```python
from build123d import *

# Parameters (mm, degrees)
BOSS_EXTRU_1_DEPTH      = 24
ESQUISSE2_W             = 2
ESQUISSE2_H             = 0.5
BOSS_EXTRU_2_DEPTH      = 3
BOSS_EXTRU_3_DEPTH      = 3
ESQUISSE6_W             = 0.6
ESQUISSE6_H             = 2
ENL_V_MAT_EXTRU_1_DEPTH = 1.5
BOSS_EXTRU_4_DEPTH      = 4
ENL_V_MAT_EXTRU_3_REACH = 29.975
ESQUISSE8_R             = 0.5
ESQUISSE9_W             = 0.5
ESQUISSE9_H             = 2
BOSS_EXTRU_5_DEPTH      = 3
ENL_V_MAT_EXTRU_2_REACH = 30.233
ESQUISSE7_R             = 0.35


with BuildPart() as part:
    # Esquisse1 → Boss.-Extru.1 (new body)
    with BuildSketch(Plane.XY):
        with BuildLine():
            Line((-3, 7), (3, 7))
            ThreePointArc((3, 7), (3.424264069, 6.824264069), (3.6, 6.4))
            Line((3.6, 6.4), (3.6, 0))
            Line((3.6, 0), (3.1, 0))
            Line((3.1, 0), (3.1, 6.4))
            ThreePointArc((3.1, 6.4), (3.070710678, 6.470710678), (3, 6.5))
            Line((3, 6.5), (-3, 6.5))
            ThreePointArc((-3, 6.5), (-3.070710678, 6.470710678), (-3.1, 6.4))
            Line((-3.1, 6.4), (-3.1, 0))
            Line((-3.1, 0), (-3.6, 0))
            Line((-3.6, 0), (-3.6, 6.4))
            ThreePointArc((-3.6, 6.4), (-3.424264069, 6.824264069), (-3, 7))
        make_face()
    extrude(amount=BOSS_EXTRU_1_DEPTH)

    # Esquisse2 → Boss.-Extru.2 (add)
    with BuildSketch(Plane(origin=(0, 0, 0), x_dir=(-1, 0, 0), z_dir=(0, 0, -1))):
        with Locations((0, 6.75)):
            Rectangle(ESQUISSE2_W, ESQUISSE2_H)
    extrude(amount=BOSS_EXTRU_2_DEPTH)

    # Esquisse5 → Boss.-Extru.3 (add)
    with BuildSketch(Plane.ZY.offset(1)):
        with BuildLine():
            Line((-0.1, 1), (-0.6, 1))
            Line((-0.6, 1), (-0.6, 6.4))
            ThreePointArc((-0.6, 6.4), (-0.424264069, 6.824264069), (0, 7))
            Line((0, 7), (0, 6.5))
            ThreePointArc((0, 6.5), (-0.070710678, 6.470710678), (-0.1, 6.4))
            Line((-0.1, 6.4), (-0.1, 1))
        make_face()
    boss_extru_3 = extrude(amount=BOSS_EXTRU_3_DEPTH)

    # Esquisse6 → Enl_v. mat.-Extru.1 (cut)
    with BuildSketch(Plane.ZY.offset(4)):
        with Locations((-0.3, 6)):
            Rectangle(ESQUISSE6_W, ESQUISSE6_H)
    enl_v_mat_extru_1 = extrude(amount=-ENL_V_MAT_EXTRU_1_DEPTH, mode=Mode.SUBTRACT)

    # Esquisse3 → Boss.-Extru.4 (add)
    with BuildSketch(Plane(origin=(0, 5, 0), x_dir=(1, 0, 0), z_dir=(0, 1, 0))):
        with BuildLine():
            Line((-4.491491227, 0.344145862), (-9.653679154, -7.028222537))
            Line((-9.653679154, -7.028222537), (-9.244103132, -7.315010755))
            Line((-9.244103132, -7.315010755), (-4.081915204, 0.057357644))
            ThreePointArc((-4.081915204, 0.057357644), (-4.046174861, 0.088701083), (-4, 0.1))
            Line((-4, 0.1), (-4, 0.6))
            ThreePointArc((-4, 0.6), (-4.277049168, 0.5322065), (-4.491491227, 0.344145862))
        make_face()
    boss_extru_4 = extrude(amount=-BOSS_EXTRU_4_DEPTH)

    # Esquisse8 → Enl_v. mat.-Extru.3 (cut, up to next)
    with BuildSketch(Plane(origin=(-3.175531513, 0, -2.223531103), x_dir=(-0.5735764363510417, 0, 0.8191520442889949), z_dir=(-0.819152044288995, 0, -0.5735764363510417)), mode=Mode.PRIVATE) as enl_v_mat_extru_3_sk1:
        with Locations((8.058237768, 3)):
            Circle(ESQUISSE8_R)
    enl_v_mat_extru_3_tool1 = extrude(enl_v_mat_extru_3_sk1.sketch, amount=-ENL_V_MAT_EXTRU_3_REACH, mode=Mode.PRIVATE) & part.part
    # Esquisse8 → Enl_v. mat.-Extru.3 (cut, up to next)
    with BuildSketch(Plane(origin=(-3.175531513, 0, -2.223531103), x_dir=(-0.5735764363510417, 0, 0.8191520442889949), z_dir=(-0.819152044288995, 0, -0.5735764363510417)), mode=Mode.PRIVATE) as enl_v_mat_extru_3_sk2:
        with BuildLine():
            Line((11.294305745, 1), (10.294305745, 1))
            ThreePointArc((10.294305745, 1), (11.058237768, 3), (10.294305745, 5))
            Line((10.294305745, 5), (11.294305745, 5))
            Line((11.294305745, 5), (11.294305745, 1))
        make_face()
    enl_v_mat_extru_3_tool2 = extrude(enl_v_mat_extru_3_sk2.sketch, amount=-ENL_V_MAT_EXTRU_3_REACH, mode=Mode.PRIVATE) & part.part
    enl_v_mat_extru_3_1 = enl_v_mat_extru_3_tool1.solids().sort_by_distance((-7.797547, 3, 4.377391))[0]
    add(enl_v_mat_extru_3_1, mode=Mode.SUBTRACT)
    enl_v_mat_extru_3_2 = enl_v_mat_extru_3_tool2.solids().sort_by_distance((-9.541925, 3, 6.868621))[0]
    add(enl_v_mat_extru_3_2, mode=Mode.SUBTRACT)
    enl_v_mat_extru_3 = enl_v_mat_extru_3_1 + enl_v_mat_extru_3_2  # Enl_v. mat.-Extru.3 as one shape, for the pattern or mirror that repeats it

    # Esquisse9 → Boss.-Extru.5 (add)
    with BuildSketch(Plane.XZ):
        with Locations((-3.35, 7.5)):
            Rectangle(ESQUISSE9_W, ESQUISSE9_H)
        with Locations((-3.35, 20.5)):
            Rectangle(ESQUISSE9_W, ESQUISSE9_H)
    boss_extru_5 = extrude(amount=BOSS_EXTRU_5_DEPTH)

    # Sym_trie1: Boss.-Extru.3, Enl_v. mat.-Extru.1, Boss.-Extru.4, Enl_v. mat.-Extru.3, Boss.-Extru.5 across plane
    add(boss_extru_3.mirror(Plane(origin=(0, 0, 0), x_dir=(0, 0, 1), z_dir=(1, 0, 0))))
    add(enl_v_mat_extru_1.mirror(Plane(origin=(0, 0, 0), x_dir=(0, 0, 1), z_dir=(1, 0, 0))), mode=Mode.SUBTRACT)
    add(boss_extru_4.mirror(Plane(origin=(0, 0, 0), x_dir=(0, 0, 1), z_dir=(1, 0, 0))))
    add(enl_v_mat_extru_3.mirror(Plane(origin=(0, 0, 0), x_dir=(0, 0, 1), z_dir=(1, 0, 0))), mode=Mode.SUBTRACT)
    add(boss_extru_5.mirror(Plane(origin=(0, 0, 0), x_dir=(0, 0, 1), z_dir=(1, 0, 0))))

    # Esquisse7 → Enl_v. mat.-Extru.2 (cut, up to next)
    with BuildSketch(Plane(origin=(3.6, 0, 0), x_dir=(0, 0, -1), z_dir=(1, 0, 0)), mode=Mode.PRIVATE) as enl_v_mat_extru_2_sk1:
        with Locations((-23, 5.5)):
            Circle(ESQUISSE7_R)
    enl_v_mat_extru_2_tool1 = extrude(enl_v_mat_extru_2_sk1.sketch, amount=-ENL_V_MAT_EXTRU_2_REACH, mode=Mode.PRIVATE) & part.part
    # Esquisse7 → Enl_v. mat.-Extru.2 (cut, up to next)
    with BuildSketch(Plane(origin=(3.6, 0, 0), x_dir=(0, 0, -1), z_dir=(1, 0, 0)), mode=Mode.PRIVATE) as enl_v_mat_extru_2_sk2:
        with BuildLine():
            Line((-24, 3.95), (-10, 3.95))
            ThreePointArc((-10, 3.95), (-9.25, 3.2), (-10, 2.45))
            Line((-10, 2.45), (-24, 2.45))
            Line((-24, 2.45), (-24, 3.95))
        make_face()
    enl_v_mat_extru_2_tool2 = extrude(enl_v_mat_extru_2_sk2.sketch, amount=-ENL_V_MAT_EXTRU_2_REACH, mode=Mode.PRIVATE) & part.part
    add(enl_v_mat_extru_2_tool1.solids().sort_by_distance((3.6, 5.5, 23))[0], mode=Mode.SUBTRACT)
    add(enl_v_mat_extru_2_tool2.solids().sort_by_distance((3.6, 3.2, 16.704515))[0], mode=Mode.SUBTRACT)


solid = part.part
```
Here's how the part is built. I have some questions about the finished solid (model axes, mm). A direction names the side the tool comes from. Coordinates: 2 decimals unless noted, no trailing zeros. Order: outer loops, then holes, each group sorted by start corner. A loop starts at its lowest first (then second) coordinate and runs counter-clockwise, first axis right, second up. Notation, with made-up numbers: M -37.75,50.5 L -25.75,50.5 A28 ccw -25.75,72.5 Z; hole C 59.25,64 d11. An arc over 180 degrees is marked long. Answer as a JSON object with one key per item and string values. Group by question number.
(1) Suppose I cut it at A-A, the plane z = 16.75. Please give me the cut outline in (x, y).
(2) Suppose I cut it at D-D, the plane y = -1.5. Please give me the cut outline in (x, z), then the cut area to 3 significant figures.
(3) Which directions (+Z, -Z, +X, -X, +Y, -Y) give clear straight access to the entire face, cutting with the end or side of a thin tool? Please do faces 4 (the face through (-6.97, 3.028, 3.195)), 5 (the face through (3.1, 2, 12)), 6 (the face through (-6.63, 3.03, 3.58)).
(4) Suppose I cut it at C-C, the plane x = 1.5. Please give me the cut outline in (y, z), then the cut area to 3 significant figures.
(5) If we mould it in two halves opening along Z, with no side actions, what happens to faces 1 (the face through (7.87, 3.15, 4.91)), 2 (the face through (6.97, 3.028, 3.195)), 3 (the face through (-6, 5, 2.4))? For each: released by +Z, released by -Z, zero draft, split by the parting line, or undercut.
(6) Suppose I cut it at B-B, the plane z = 23. Please give me the cut outline in (x, y).
(7) I need wall thicknesses on probe 1 along Y at (x, z) = (3.3, 23); probe 2 along Y at (x, z) = (3.45, 23); probe 3 along Z at (x, y) = (3.5, -2). Which ranges of each line are inside material? Lowest first, please.
(8) For pin 1 (0.6 mm diameter, centred on y = 7, z = -1, fed in from +X); pin 2 (2 mm diameter, centred on y = 4.5, z = 9.5, fed in from -X); pin 3 (4.5 mm diameter, centred on y = 4, z = 11.5, fed in from +X); pin 4 (4 mm diameter, centred on x = 5, z = 15.5, fed in from +Y), each with a flat end and sliding along its axis, tell me the tip position at first contact or that it passes through.
Values found:
{
 "1": {"outline": "M -3.6,0 L -3.1,0 L -3.1,6.4 A0.1 cw -3,6.5 L 3,6.5 A0.1 cw 3.1,6.4 L 3.1,3.95 L 3.6,3.95 L 3.6,6.4 A0.6 ccw 3,7 L -3,7 A0.6 ccw -3.6,6.4 Z; M 3.1,0 L 3.6,0 L 3.6,2.45 L 3.1,2.45 Z"},
 "2": {"outline": "M -3.6,6.5 L -3.1,6.5 L -3.1,8.5 L -3.6,8.5 Z; M -3.6,19.5 L -3.1,19.5 L -3.1,21.5 L -3.6,21.5 Z; M 3.1,6.5 L 3.6,6.5 L 3.6,8.5 L 3.1,8.5 Z; M 3.1,19.5 L 3.6,19.5 L 3.6,21.5 L 3.1,21.5 Z", "area": "4.00 mm^2"},
 "3": {"face 4": "-Z, -X, +Y, -Y", "face 5": "+Z, -Y", "face 6": "+Z, +Y, -Y"},
 "4": {"outline": "M 1,-0.6 L 6.4,-0.6 A0.6 ccw 7,0 L 7,24 L 6.5,24 L 6.5,0 A0.1 cw 6.4,-0.1 L 1,-0.1 Z", "area": "15.0 mm^2"},
 "5": {"face 1": "undercut", "face 2": "released by -Z", "face 3": "zero draft"},
 "6": {"outline": "M -3.6,0 L -3.1,0 L -3.1,6.4 A0.1 cw -3,6.5 L 3,6.5 A0.1 cw 3.1,6.4 L 3.1,5.85 L 3.6,5.85 L 3.6,6.4 A0.6 ccw 3,7 L -3,7 A0.6 ccw -3.6,6.4 Z; M 3.1,0 L 3.6,0 L 3.6,2.45 L 3.1,2.45 Z; M 3.1,3.95 L 3.6,3.95 L 3.6,5.15 L 3.1,5.15 Z"},
 "7": {"probe 1": "y = 0 to 2.45, 3.95 to 5.15, 5.85 to 6.92", "probe 2": "y = 0 to 2.45, 3.95 to 5.15, 5.85 to 6.8", "probe 3": "z = 6.5 to 8.5, 19.5 to 21.5"},
 "8": {"pin 1": "stops at x = 1", "pin 2": "stops at x = -3.6", "pin 3": "stops at x = 3.6", "pin 4": "stops at y = 7"}
}
